Read the model definition and answer for the solid it produces. Units are mm, in the model's axes. A direction names the side the tool comes from. Coordinates: 2 decimals unless noted, no trailing zeros. Loops run counter-clockwise (first coordinate to the right, second up) from the corner with the lowest first, then second, coordinate; pieces in that order, holes last. Notation, with made-up numbers: (79.5, -25.75) - (106.5, -25.75) arc R24 ccw to (106.5, -4.75) - close; hole circle Ø3 at (87, 47). An arc over 180 degrees is marked (long way). Use one line per item in the form item = value.
from build123d import *

# Parameters (mm, degrees)
BOSS_EXTRUDE1_DEPTH         = 5
TAP_DRILL_FOR_M4X0_7_TAP1_D = 4
BOSS_EXTRUDE2_DEPTH         = 20.6
CIRPATTERN1_COUNT           = 4


with BuildPart() as part:
    # Sketch1 → Boss-Extrude1 (new body)
    with BuildSketch(Plane(origin=(0, 0, 0), x_dir=(1, 0, 0), z_dir=(0, 1, 0))):
        with BuildLine():
            Line((6, 95), (11.656854249, 95))
            ThreePointArc((11.656854249, 95), (12.039537682, 94.923879533), (12.363961031, 94.707106781))
            Line((12.363961031, 94.707106781), (32.538709783, 74.532358029))
            ThreePointArc((32.538709783, 74.532358029), (33.362638794, 74.138893326), (34.250764856, 74.350802705))
            ThreePointArc((34.250764856, 74.350802705), (50, 79), (65.749235144, 74.350802705))
            ThreePointArc((65.749235144, 74.350802705), (66.637361206, 74.138893326), (67.461290217, 74.532358029))
            Line((67.461290217, 74.532358029), (87.636038969, 94.707106781))
            ThreePointArc((87.636038969, 94.707106781), (87.960462318, 94.923879533), (88.343145751, 95))
            Line((88.343145751, 95), (94, 95))
            ThreePointArc((94, 95), (94.707106781, 94.707106781), (95, 94))
            Line((95, 94), (95, 88.343145751))
            ThreePointArc((95, 88.343145751), (94.923879533, 87.960462318), (94.707106781, 87.636038969))
            Line((94.707106781, 87.636038969), (74.532358029, 67.461290217))
            ThreePointArc((74.532358029, 67.461290217), (74.138893326, 66.637361206), (74.350802705, 65.749235144))
            ThreePointArc((74.350802705, 65.749235144), (79, 50), (74.350802705, 34.250764856))
            ThreePointArc((74.350802705, 34.250764856), (74.138893326, 33.362638794), (74.532358029, 32.538709783))
            Line((74.532358029, 32.538709783), (94.707106781, 12.363961031))
            ThreePointArc((94.707106781, 12.363961031), (94.923879533, 12.039537682), (95, 11.656854249))
            Line((95, 11.656854249), (95, 6))
            ThreePointArc((95, 6), (94.707106781, 5.292893219), (94, 5))
            Line((94, 5), (88.343145751, 5))
            ThreePointArc((88.343145751, 5), (87.960462318, 5.076120467), (87.636038969, 5.292893219))
            Line((87.636038969, 5.292893219), (67.461290217, 25.467641971))
            ThreePointArc((67.461290217, 25.467641971), (66.637361206, 25.861106674), (65.749235144, 25.649197295))
            ThreePointArc((65.749235144, 25.649197295), (50, 21), (34.250764856, 25.649197295))
            ThreePointArc((34.250764856, 25.649197295), (33.362638794, 25.861106674), (32.538709783, 25.467641971))
            Line((32.538709783, 25.467641971), (12.363961031, 5.292893219))
            ThreePointArc((12.363961031, 5.292893219), (12.039537682, 5.076120467), (11.656854249, 5))
            Line((11.656854249, 5), (6, 5))
            ThreePointArc((6, 5), (5.292893219, 5.292893219), (5, 6))
            Line((5, 6), (5, 11.656854249))
            ThreePointArc((5, 11.656854249), (5.076120467, 12.039537682), (5.292893219, 12.363961031))
            Line((5.292893219, 12.363961031), (25.467641971, 32.538709783))
            ThreePointArc((25.467641971, 32.538709783), (25.861106674, 33.362638794), (25.649197295, 34.250764856))
            ThreePointArc((25.649197295, 34.250764856), (21, 50), (25.649197295, 65.749235144))
            ThreePointArc((25.649197295, 65.749235144), (25.861106674, 66.637361206), (25.467641971, 67.461290217))
            Line((25.467641971, 67.461290217), (5.292893219, 87.636038969))
            ThreePointArc((5.292893219, 87.636038969), (5.076120467, 87.960462318), (5, 88.343145751))
            Line((5, 88.343145751), (5, 94))
            ThreePointArc((5, 94), (5.292893219, 94.707106781), (6, 95))
        make_face()
        with BuildLine():
            Line((72.980970389, 58.838834765), (58.838834765, 72.980970389))
            ThreePointArc((58.838834765, 72.980970389), (32.589514654, 67.410485346), (27.019029611, 41.161165235))
            Line((27.019029611, 41.161165235), (41.161165235, 27.019029611))
            ThreePointArc((41.161165235, 27.019029611), (67.410485346, 32.589514654), (72.980970389, 58.838834765))
        make_face(mode=Mode.SUBTRACT)
    extrude(amount=BOSS_EXTRUDE1_DEPTH)

    # Tap Drill for M4x0.7 Tap1 (through all)
    with Locations(Plane(origin=(31.749573978, 5, -31.749573978), x_dir=(0, 0, 1), z_dir=(0, 1, 0))):
        with Locations((0, 0), (-36.500852044, 36.500852044)):
            Hole(TAP_DRILL_FOR_M4X0_7_TAP1_D / 2)

    # Sketch6 → Boss-Extrude2 (add)
    with BuildSketch(Plane(origin=(0, 5, 0), x_dir=(1, 0, 0), z_dir=(0, 1, 0))):
        with BuildLine():
            Line((6, 95), (11.656854249, 95))
            ThreePointArc((11.656854249, 95), (12.039537682, 94.923879533), (12.363961031, 94.707106781))
            Line((12.363961031, 94.707106781), (12.707106781, 94.363961031))
            ThreePointArc((12.707106781, 94.363961031), (12.923879533, 94.039537682), (13, 93.656854249))
            Line((13, 93.656854249), (13, 88))
            ThreePointArc((13, 88), (12.707106781, 87.292893219), (12, 87))
            Line((12, 87), (6.343145751, 87))
            ThreePointArc((6.343145751, 87), (5.960462318, 87.076120467), (5.636038969, 87.292893219))
            Line((5.636038969, 87.292893219), (5.292893219, 87.636038969))
            ThreePointArc((5.292893219, 87.636038969), (5.076120467, 87.960462318), (5, 88.343145751))
            Line((5, 88.343145751), (5, 94))
            ThreePointArc((5, 94), (5.292893219, 94.707106781), (6, 95))
        make_face()
    boss_extrude2 = extrude(amount=BOSS_EXTRUDE2_DEPTH)

    # Sketch9 → Tap Drill for M2x0.4 Tap1 (revolve, cut)
    with BuildSketch(Plane(origin=(9, 25.6, -91), x_dir=(0, 0, 1), z_dir=(1, 0, 0))):
        Polygon((0, 0), (0, 4.600860619), (1, 4), (1, 0), align=None)
    tap_drill_for_m2x0_4_tap1 = revolve(axis=Axis((9, 31.95, -91), (0, -1, 0)), mode=Mode.SUBTRACT)

    # CirPattern1: Boss-Extrude2, Tap Drill for M2x0.4 Tap1 ×4 about axis
    cirpattern1_axis = Axis((50, 0, -50), (0, 1, 0))
    for i in range(1, CIRPATTERN1_COUNT):
        add(boss_extrude2.rotate(cirpattern1_axis, i * 360 / CIRPATTERN1_COUNT))
        add(tap_drill_for_m2x0_4_tap1.rotate(cirpattern1_axis, i * 360 / CIRPATTERN1_COUNT), mode=Mode.SUBTRACT)


solid = part.part
Item 1: Which of the six approach directions +Z, -Z, +X, -X, +Y, -Y give full straight-line access (tool end or side, diameter ignored) to faces 1 (the flat face through (86.16, 4.21, -79.09)), 2 (the flat face through (13.84, 4.21, -20.91)), 3 (the cylindrical face through (9, 24, -92))?
Results below:
face_1 = +X, +Y, -Y
face_2 = -X, +Y, -Y
face_3 = +Y
Item 2: The part is cut by section A-A on x = 54. Give the vertices of the cut face in (y, z).
Results below:
outline = (0, -78.72) - (5, -78.72) - (5, -74.3) - (0, -74.3) - close; (0, -25.7) - (5, -25.7) - (5, -21.28) - (0, -21.28) - close
Item 3: The part is cut by section C-C on z = -40. Give the vertices of the cut face in (x, y).
Results below:
outline = (22.78, 0) - (28.18, 0) - (28.18, 5) - (22.78, 5) - close; (72.5, 0) - (77.22, 0) - (77.22, 5) - (72.5, 5) - close
Item 4: Each of these flat-tipped pins is pushed along its axis until it touches: P1, Ø6.5, axis at x = 31.75, z = -31.75, coming from the +Y side; P2, Ø1.6, axis at x = 91, z = -9, coming from the +Y side; P3, Ø10, axis at y = 5, z = -22, coming from the -X side; P4, Ø12, axis at x = 67, y = 11.5, coming from the -Z side. Where does it stop, or does it pass through?
Results below:
P1 = 5
P2 = 21.48
P3 = 9.93
P4 = through
Item 5: The part is cut by section D-D on z = -23. Give the vertices of the cut face in (x, y).
Results below:
outline = (15.93, 0) - (30.07, 0) - (30.07, 5) - (15.93, 5) - close; (39.42, 0) - (60.58, 0) - (60.58, 5) - (39.42, 5) - close; (69.93, 0) - (84.07, 0) - (84.07, 5) - (69.93, 5) - close
Item 6: The part is cut by section B-B on y = 23.25. Count the separate pieces of the cut face and the enclosed holes in it, plus the area to 3 significant figures.
Results below:
separate_pieces = 4
enclosed_holes = 4
area = 238 mm²
Item 7: Find the intervals of material crossed by L1, parallel to Z at x = 91, y = 24.1; L2, parallel to Z at x = 50.5, y = 2; L3, parallel to X at y = 24.45, z = -91, in increasing order.
Results below:
L1 = -95 to -92, -90 to -87, -13 to -10, -8 to -5
L2 = -79 to -74.62, -25.38 to -21
L3 = 5 to 8, 10 to 13, 87 to 90, 92 to 95
Item 8: For a pull along X with two mould halves and no side action, classify faces 4 (the flat face through (9, 15, -13)), 5 (the flat face through (79.09, 4.21, -13.84)), 6 (the cylindrical face through (79, 2, -50)) as +X half, -X half, draft (parallel to the pull), parting line (faces both ways), or undercut.
Results below:
face_4 = draft
face_5 = undercut
face_6 = +X half
